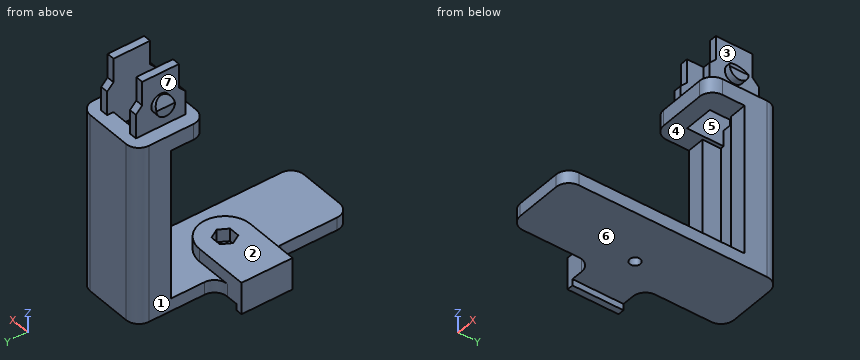
```python
from build123d import *

# Parameters (mm, degrees)
SKETCH1_R           = 1.65
BOSS_EXTRUDE1_DEPTH = 75
CUT_EXTRUDE3_REACH  = 90.246
CUT_EXTRUDE4_REACH  = 85.882
SKETCH5_W           = 9.2
SKETCH5_H           = 11.5
SKETCH6_W           = 11.5
SKETCH6_H           = 11.5
CUT_EXTRUDE5_DEPTH  = 47
SKETCH7_W           = 30.25
SKETCH7_H           = 67
CUT_EXTRUDE6_DEPTH  = 2
CUT_EXTRUDE7_DEPTH  = 4
SKETCH9_W           = 17
SKETCH9_H           = 22
SKETCH9_R           = 2.9
CUT_EXTRUDE8_DEPTH  = 4.25
CUT_EXTRUDE9_START  = -4.25
SKETCH10_W          = 17
SKETCH10_H          = 22
SKETCH10_R          = 2.9
CUT_EXTRUDE9_DEPTH  = 4.25
CUT_EXTRUDE10_DEPTH = 17
CUT_EXTRUDE11_START = -18.25
CUT_EXTRUDE11_DEPTH = 14
CUT_EXTRUDE12_REACH = 103.995


with BuildPart() as part:
    # Sketch1 → Boss-Extrude1 (new body)
    with BuildSketch(Plane.XY):
        with BuildLine():
            Line((-17, -8), (-17, 8))
            Line((-17, 8), (-11.25, 8))
            ThreePointArc((-11.25, 8), (-8.421572875, 9.171572875), (-7.25, 12))
            Line((-7.25, 12), (-7.25, 29.5))
            ThreePointArc((-7.25, 29.5), (-6.078427125, 32.328427125), (-3.25, 33.5))
            Line((-3.25, 33.5), (11.25, 33.5))
            ThreePointArc((11.25, 33.5), (14.078427125, 32.328427125), (15.25, 29.5))
            Line((15.25, 29.5), (15.25, -29.5))
            ThreePointArc((15.25, -29.5), (14.078427125, -32.328427125), (11.25, -33.5))
            Line((11.25, -33.5), (-3.25, -33.5))
            ThreePointArc((-3.25, -33.5), (-6.078427125, -32.328427125), (-7.25, -29.5))
            Line((-7.25, -29.5), (-7.25, -12))
            ThreePointArc((-7.25, -12), (-8.421572875, -9.171572875), (-11.25, -8))
            Line((-11.25, -8), (-17, -8))
        make_face()
        Circle(SKETCH1_R, mode=Mode.SUBTRACT)
    extrude(amount=BOSS_EXTRUDE1_DEPTH)

    # Cut-Extrude3: up to this face of the body (flat: up to its plane)
    cut_extrude3_end = Plane(part.part.faces().sort_by_distance((-17, 0, 37.5))[0])
    # Sketch4 → Cut-Extrude3 (cut, up to the picked face)
    with BuildSketch(Plane(origin=(15.25, 0, 0), x_dir=(0, 0, -1), z_dir=(1, 0, 0)), mode=Mode.PRIVATE) as cut_extrude3_sk1:
        Polygon((-75, 11.5), (-75, -33.5), (-6, -33.5), (-6, -8), (-10, -8), (-10, 8), (-6, 8), (-6, 22.5), (-53, 22.5), (-53, 11.5), align=None)
    cut_extrude3_tool1 = split(extrude(cut_extrude3_sk1.sketch, amount=-CUT_EXTRUDE3_REACH, mode=Mode.PRIVATE), bisect_by=cut_extrude3_end, keep=Keep.BOTH, mode=Mode.PRIVATE)
    add(cut_extrude3_tool1.solids().sort_by(Axis((15.25, -7.129286, 39.486228), (-1, 0, 0)))[0], mode=Mode.SUBTRACT)

    # Cut-Extrude4: up to this face of the body (flat: up to its plane)
    cut_extrude4_end = Plane(part.part.faces().sort_by_distance((3.873526685, 15.183797252, 6))[0])
    # Sketch5 → Cut-Extrude4 (cut, up to the picked face)
    with BuildSketch(Plane.XY.offset(75), mode=Mode.PRIVATE) as cut_extrude4_sk1:
        with Locations((4, 22.5)):
            Rectangle(SKETCH5_W, SKETCH5_H)
    cut_extrude4_tool1 = split(extrude(cut_extrude4_sk1.sketch, amount=-CUT_EXTRUDE4_REACH, mode=Mode.PRIVATE), bisect_by=cut_extrude4_end, keep=Keep.BOTH, mode=Mode.PRIVATE)
    # Sketch5 → Cut-Extrude4 (cut, up to the picked face)
    with BuildSketch(Plane.XY.offset(75), mode=Mode.PRIVATE) as cut_extrude4_sk2:
        with BuildLine():
            Line((11.25, 11.5), (15.25, 11.5))
            Line((15.25, 11.5), (15.25, 15.5))
            ThreePointArc((15.25, 15.5), (14.078427125, 12.671572875), (11.25, 11.5))
        make_face()
    cut_extrude4_tool2 = split(extrude(cut_extrude4_sk2.sketch, amount=-CUT_EXTRUDE4_REACH, mode=Mode.PRIVATE), bisect_by=cut_extrude4_end, keep=Keep.BOTH, mode=Mode.PRIVATE)
    # Sketch5 → Cut-Extrude4 (cut, up to the picked face)
    with BuildSketch(Plane.XY.offset(75), mode=Mode.PRIVATE) as cut_extrude4_sk3:
        with BuildLine():
            Line((-7.281373033, 11.5), (-3.25, 11.5))
            ThreePointArc((-3.25, 11.5), (-6.078427125, 12.671572875), (-7.25, 15.5))
            Line((-7.25, 15.5), (-7.25, 12))
            ThreePointArc((-7.25, 12), (-7.257850963, 11.74950835), (-7.281373033, 11.5))
        make_face()
    cut_extrude4_tool3 = split(extrude(cut_extrude4_sk3.sketch, amount=-CUT_EXTRUDE4_REACH, mode=Mode.PRIVATE), bisect_by=cut_extrude4_end, keep=Keep.BOTH, mode=Mode.PRIVATE)
    # Sketch5 → Cut-Extrude4 (cut, up to the picked face)
    with BuildSketch(Plane.XY.offset(75), mode=Mode.PRIVATE) as cut_extrude4_sk4:
        with BuildLine():
            Line((0, 8), (15.25, 8))
            Line((15.25, 8), (15.25, -8))
            Line((15.25, -8), (0, -8))
            ThreePointArc((0, -8), (8, 0), (0, 8))
        make_face()
    cut_extrude4_tool4 = split(extrude(cut_extrude4_sk4.sketch, amount=-CUT_EXTRUDE4_REACH, mode=Mode.PRIVATE), bisect_by=cut_extrude4_end, keep=Keep.BOTH, mode=Mode.PRIVATE)
    add(cut_extrude4_tool1.solids().sort_by(Axis((4, 22.5, 75), (0, 0, -1)))[0], mode=Mode.SUBTRACT)
    add(cut_extrude4_tool2.solids().sort_by(Axis((14.356528, 12.393472, 75), (0, 0, -1)))[0], mode=Mode.SUBTRACT)
    add(cut_extrude4_tool3.solids().sort_by(Axis((-6.357899, 12.392305, 75), (0, 0, -1)))[0], mode=Mode.SUBTRACT)
    add(cut_extrude4_tool4.solids().sort_by(Axis((10.588812, 0, 75), (0, 0, -1)))[0], mode=Mode.SUBTRACT)

    # Sketch6 → Cut-Extrude5 (cut)
    with BuildSketch(Plane.XY.offset(6)):
        with Locations((4, 22.5)):
            Rectangle(SKETCH6_W, SKETCH6_H)
    extrude(amount=CUT_EXTRUDE5_DEPTH, mode=Mode.SUBTRACT)

    # Sketch7 → Cut-Extrude6 (cut)
    with BuildSketch(Plane(origin=(0, 0, 0), x_dir=(-1, 0, 0), z_dir=(0, 0, -1))):
        with Locations((-0.125, 0)):
            Rectangle(SKETCH7_W, SKETCH7_H)
    extrude(amount=-CUT_EXTRUDE6_DEPTH, mode=Mode.SUBTRACT)

    # Sketch8 → Cut-Extrude7 (cut)
    with BuildSketch(Plane.XY.offset(10)):
        Polygon((3.348631561, 0), (1.674315781, 2.9), (-1.674315781, 2.9), (-3.348631561, 0), (-1.674315781, -2.9), (1.674315781, -2.9), align=None)
    extrude(amount=-CUT_EXTRUDE7_DEPTH, mode=Mode.SUBTRACT)

    # Sketch9 → Cut-Extrude8 (cut)
    with BuildSketch(Plane(origin=(15.25, 0, 0), x_dir=(0, 0, -1), z_dir=(1, 0, 0))):
        with Locations((-66.5, 22.5)):
            Rectangle(SKETCH9_W, SKETCH9_H)
        with Locations(Location((-65.5, 22.5, 0), (0, 0, 90))):
            Circle(SKETCH9_R, mode=Mode.SUBTRACT)
    extrude(amount=-CUT_EXTRUDE8_DEPTH, mode=Mode.SUBTRACT)

    # Sketch10 → Cut-Extrude9 (cut)
    with BuildSketch(Plane.ZY.offset(7.25).offset(CUT_EXTRUDE9_START)):
        with Locations((66.5, 22.5)):
            Rectangle(SKETCH10_W, SKETCH10_H)
        with Locations(Location((65.5, 22.5, 0), (0, 0, 90))):
            Circle(SKETCH10_R, mode=Mode.SUBTRACT)
    extrude(amount=CUT_EXTRUDE9_DEPTH, mode=Mode.SUBTRACT)

    # Sketch11 → Cut-Extrude10 (cut)
    with BuildSketch(Plane.XY.offset(75)):
        Polygon((-7.25, 14.75), (-7.25, 11.5), (15.25, 11.5), (15.25, 14.75), (8.6, 14.75), (8.6, 30.25), (15.25, 30.25), (15.25, 33.5), (-7.25, 33.5), (-7.25, 30.25), (-0.6, 30.25), (-0.6, 14.75), align=None)
    extrude(amount=-CUT_EXTRUDE10_DEPTH, mode=Mode.SUBTRACT)

    # Sketch12 → Cut-Extrude11 (cut)
    with BuildSketch(Plane.ZY.offset(7.25).offset(CUT_EXTRUDE11_START)):
        Polygon((65.5, 30.25), (67.5, 28.25), (75, 28.25), (75, 30.25), align=None)
        Polygon((65.5, 14.75), (67.5, 16.75), (75, 16.75), (75, 14.75), align=None)
    extrude(amount=CUT_EXTRUDE11_DEPTH, mode=Mode.SUBTRACT)

    # Cut-Extrude12: up to this face of the body (flat: up to its plane)
    cut_extrude12_end = Plane(part.part.faces().sort_by_distance((4, 11.5, 55.5))[0])
    # Sketch13 → Cut-Extrude12 (cut, up to the picked face)
    with BuildSketch(Plane(origin=(0, 33.5, 0), x_dir=(1, 0, 0), z_dir=(0, 1, 0)), mode=Mode.PRIVATE) as cut_extrude12_sk1:
        Polygon((-5.1, -65.5), (-3.5, -68.4), (-7.25, -68.4), (-7.25, -62.6), (-5.125, -62.6), align=None)
    cut_extrude12_tool1 = split(extrude(cut_extrude12_sk1.sketch, amount=-CUT_EXTRUDE12_REACH, mode=Mode.PRIVATE), bisect_by=cut_extrude12_end, keep=Keep.BOTH, mode=Mode.PRIVATE)
    # Sketch13 → Cut-Extrude12 (cut, up to the picked face)
    with BuildSketch(Plane(origin=(0, 33.5, 0), x_dir=(1, 0, 0), z_dir=(0, 1, 0)), mode=Mode.PRIVATE) as cut_extrude12_sk2:
        Polygon((13.1, -65.5), (11.5, -68.4), (15.25, -68.4), (15.25, -62.6), (13.125, -62.6), align=None)
    cut_extrude12_tool2 = split(extrude(cut_extrude12_sk2.sketch, amount=-CUT_EXTRUDE12_REACH, mode=Mode.PRIVATE), bisect_by=cut_extrude12_end, keep=Keep.BOTH, mode=Mode.PRIVATE)
    add(cut_extrude12_tool1.solids().sort_by(Axis((-5.924713, 33.5, 65.808763), (0, -1, 0)))[0], mode=Mode.SUBTRACT)
    add(cut_extrude12_tool2.solids().sort_by(Axis((13.924713, 33.5, 65.808763), (0, -1, 0)))[0], mode=Mode.SUBTRACT)


solid = part.part
```
Geometry: final body of the model. Coordinates: model frame, mm. Face numbers are marked on the shaded views. A direction names the side the tool comes from. Coordinates: 2 decimals unless noted, no trailing zeros. Order: outer loops, then holes, each group sorted by start corner. A loop starts at its lowest first (then second) coordinate and runs counter-clockwise, first axis right, second up. Notation, with made-up numbers: (63.25, -31.5) - (99.25, -31.5) arc R29 ccw to (99.25, 5.5) - close; hole circle Ø10 at (-10, 63.25). An arc over 180 degrees is marked (long way). Return JSON: item names as keys, results as strings. Group by question number.
1. Set-up query: the marked faces 1, 2, 3 and 4. Return all of +Z, -Z, +X, -X, +Y, -Y with unobstructed straight access to the full face (end or side cutting, diameter ignored); none if empty.
2. Material intervals for line 1 along X through (y, z) = (0, 3.25); line 2 along Y through (x, z) = (0, 4.3); line 3 along Z through (x, y) = (-6.5, 21.5), sorted ascending. Write a range as [from, to].
3. Cut plane A-A (z = 55). Output: boundary loops of the cut face in (x, y).
4. Pin query (flat end, axial travel): pin 1 (12 mm diameter, centred on y = 12.5, z = 61, fed in from +X); pin 2 (12.5 mm diameter, centred on y = 19, z = 67.5, fed in from +X) (3 decimals); pin 3 (4 mm diameter, centred on x = 0, y = 0, fed in from +Z); pin 4 (13 mm diameter, centred on x = -4, y = -2.5, fed in from +Z). Return the tip coordinate at first contact, or that it passes through.
5. Cut plane B-B (x = 4.5). Output: boundary loops of the cut face in (y, z).
6. Pull-direction query (Z, two-part tool) for the marked faces 5, 6 and 7; classes: pulls with the +Z half, pulls with the -Z half, needs draft (parallel to the pull), parting line crosses it, or undercut.
7. Cut plane C-C (z = 47). Output: boundary loops of the cut face in (x, y), plus the area to 3 significant figures.
Resolved:
{
 "1": {"face 1": "+Z, -Z, -X, +Y", "face 2": "+Z, +X, -X, -Y", "face 3": "+X", "face 4": "-Y"},
 "2": {"line 1": "x = [-17, -1.65], [1.65, 15.25]", "line 2": "y = [-33.5, -1.65], [1.65, 33.5]", "line 3": "z = [2, 6], [53, 58]"},
 "3": {"outline": "(-7.25, 15.5) arc R4 ccw to (-3.25, 11.5) - (11.25, 11.5) arc R4 ccw to (15.25, 15.5) - (15.25, 29.5) arc R4 ccw to (11.25, 33.5) - (-3.25, 33.5) arc R4 ccw to (-7.25, 29.5) - close; hole (-0.6, 16.75) - (8.6, 16.75) - (8.6, 28.25) - (-0.6, 28.25) - close"},
 "4": {"pin 1": "stops at x = 15.25", "pin 2": "stops at x = 13.125", "pin 3": "stops at z = 6", "pin 4": "stops at z = 10"},
 "5": {"outline": "(-33.5, 2) - (33.5, 2) - (33.5, 58) - (28.25, 58) - (28.25, 6) - (6.61, 6) - (6.61, 10) - (-6.61, 10) - (-6.61, 6) - (-33.5, 6) - close; (11.5, 53) - (16.75, 53) - (16.75, 58) - (11.5, 58) - close"},
 "6": {"face 5": "needs draft", "face 6": "pulls with the -Z half", "face 7": "undercut"},
 "7": {"outline": "(-7.25, 22.5) - (-1.75, 22.5) - (-1.75, 28.25) - (9.75, 28.25) - (9.75, 22.5) - (15.25, 22.5) - (15.25, 29.5) arc R4 ccw to (11.25, 33.5) - (-3.25, 33.5) arc R4 ccw to (-7.25, 29.5) - close", "area": "175 mm²"}
}
